```python
from build123d import *

# Parameters (mm, degrees)
PAD_DEPTH    = 50
SKETCH_R     = 5
SKETCH_R_2   = 6.604591
SKETCH_W     = 68
SKETCH_H     = 5
POCKET_DEPTH = 50.001


with BuildPart() as part:
    # Sketch001 → Pad (new body)
    with BuildSketch(Plane.XY):
        Polygon((21.658416, -142.396888), (380.553462, 564.152424), (289.232679, 778.86121), (108.359877, 882.789603), (-104.030099, 786.198474), (-233.87883, 4.433233), align=None)
    extrude(amount=-PAD_DEPTH)

    # Sketch (on Face7 of Pad) → Pocket (cut, through all)
    with BuildSketch(Plane.XY):
        with Locations((0, 600)):
            Circle(SKETCH_R)
        with Locations((58.588821, 532.512666)):
            Circle(SKETCH_R)
        with Locations((111.61367, 496.881813)):
            Circle(SKETCH_R)
        with Locations((152.341802, 434.193515)):
            Circle(SKETCH_R)
        with Locations((184.96974, 376.321267)):
            Circle(SKETCH_R)
        with Locations((-31.108797, 715.687506)):
            Circle(SKETCH_R_2)
        with Locations((-61.54211, 721.87355)):
            Circle(SKETCH_R_2)
        with Locations((24, -2.5)):
            Rectangle(SKETCH_W, SKETCH_H)
    extrude(amount=-POCKET_DEPTH, mode=Mode.SUBTRACT)


solid = part.part
```
For this review, take the finished solid that the model builds, in its own axes (mm). A direction names the side the tool comes from. Round coordinates to 2 decimals unless told otherwise and drop trailing zeros. Write each loop counter-clockwise with the first axis right and the second up, starting at its lowest first coordinate (ties: lowest second). Pieces come first, ordered by that corner, then holes. Notation, with made-up numbers: (26, 81.25) -> (60, 81.25) arc R10 cw to (60, 89.25) -> close; hole circle Ø6 at (16, 68.25). An arc over 180 degrees is marked (long way). Use one line per item in the form item = value.
Q1. Clearance check with flat-ended pins moving along their axes: pin 1 Ø2.5 at (y, z) = (-2.5, -31.5) entering from +X; pin 2 Ø10 at (x, z) = (134, -36.5) entering from -Y; pin 3 Ø1.5 at (x, z) = (131, -20) entering from -Y. State where each tip first meets the part, or that it passes through.
Resolved:
pin_1 = 93.35
pin_2 = 68.92
pin_3 = 71.39
Q2. Consider section A-A (x = 44). State the section outline as (y, z) points, then the cut area to 3 significant figures.
Resolved:
outline = (-98.41, -50) -> (-5, -50) -> (-5, 0) -> (-98.41, 0) -> close; (0, -50) -> (853.52, -50) -> (853.52, 0) -> (0, 0) -> close
area = 47,300 mm²
Q3. To check wall thickness, follow probe 1 along Y at (x, z) = (56, -31); probe 2 along Y at (x, z) = (16.5, -42.5); probe 3 along X at (y, z) = (268.5, -28.5). State the ranges of each line that lie inside material, in increasing order. Write a range as from..to.
Resolved:
probe_1 = -74.79..-5, 0..528.24, 536.79..858.98
probe_2 = -139.43..-5, 0..841.01
probe_3 = -190.02..230.38
Q4. Consider section B-B (z = -35.5). State how many separate pieces and enclosed holes the cut face has, then the cut area to 3 significant figures.
Resolved:
separate_pieces = 1
enclosed_holes = 8
area = 381,000 mm²
Q5. The part is to be moulded in two halves that separate along Y. For faces 1 (the flat face through (69, 377, -50)), 2 (the flat face through (24, 0, -25)), 3 (the flat face through (3.65, 835.17, -24.65)), say which applies: released by +Y, released by -Y, zero draft, split by the parting line, or undercut.
Resolved:
face_1 = zero draft
face_2 = undercut
face_3 = released by +Y
Q6. Consider section C-C (x = -79). State the section outline as (y, z) points, then the cut area to 3 significant figures.
Resolved:
outline = (-84.56, -50) -> (797.58, -50) -> (797.58, 0) -> (-84.56, 0) -> close
area = 44,100 mm²
Q7. Consider section D-D (x = 210). State the section outline as (y, z) points, then the cut area to 3 significant figures.
Resolved:
outline = (228.39, -50) -> (824.39, -50) -> (824.39, 0) -> (228.39, 0) -> close
area = 29,800 mm²
Q8. Machinability: for faces 4 (the flat face through (24, -5, -25)), 5 (the flat face through (69, 377, 0)), which of the approach directions +Z, -Z, +X, -X, +Y, -Y give a long, thin tool a straight path to every point of the face, cutting with its end or side? Answer none if there is none.
Resolved:
face_4 = +Z, -Z
face_5 = +Z, +X, -X, +Y, -Y
